Autodesk Inventor part; units mm, degrees
ref_plane "YZ Plane" through (0, 0, 0) normal (1, 0, 0) x (0, 1, 0)
ref_plane "XZ Plane" through (0, 0, 0) normal (0, 1, 0) x (-1, 0, 0)
ref_plane "XY Plane" through (0, 0, 0) normal (0, 0, 1) x (1, 0, 0)
sketch "Sketch1" plane through (0, 0, 0) normal (1, 0, 0) x (0, 1, 0)
  line L0 (64.7557, 308.0174) -> (-36.8443, 308.0174)
  line L1 (-36.8443, 308.0174) -> (-36.8443, -314.2826)
  line L2 (-36.8443, -314.2826) -> (64.7557, -314.2826)
  line L3 (64.7557, -314.2826) -> (64.7557, 308.0174)
  dimension "d2" = 622.3
  dimension "d3" = 101.6
extrude "Board" add sketch "Sketch1" along normal blind 19.05
sketch "Sketch8" plane through (19.05, 0, 0) normal (1, 0, 0) x (0, 0, -1)
  line L0 (-308.0174, 55.2307) -> (314.2826, 55.2307)
  line L1 (314.2826, 55.2307) -> (314.2826, 45.7057)
  line L2 (314.2826, 45.7057) -> (-308.0174, 45.7057)
  line L3 (-308.0174, 45.7057) -> (-308.0174, 55.2307)
  line L4 (-308.0174, 64.7557) -> (-308.0174, -36.8443)
  line L5 (314.2826, -36.8443) -> (314.2826, 64.7557)
  line L6 (314.2826, 64.7557) -> (-308.0174, 64.7557)
  point P0 (0, 0)
  dimension "d22" = 9.525
  dimension "d23" = 9.525
extrude "Lenghtwise Dado for Base" cut sketch "Sketch8" against normal blind 9.525 contours L0 L1 L2 L3
sketch "Sketch 9" plane through (0, 64.7557, 308.0174) normal (0, 1, 0) x (1, 0, 0)
  line L0 (19.05, 168.275) -> (9.525, 168.275)
  line L1 (9.525, 168.275) -> (9.525, 622.3)
  line L2 (9.525, 622.3) -> (19.05, 622.3)
  line L3 (19.05, 622.3) -> (19.05, 168.275)
  line L4 (19.05, 622.3) -> (19.05, 0)
  line L5 (0, 622.3) -> (19.05, 622.3)
  point P0 (0, 308.0174)
  dimension "d26" = 454.025
  dimension "d27" = 9.525
extrude "Lengthwise stop dado for Sides" cut sketch "Sketch 9" against normal blind 9.525
sketch "Sketch12" plane through (19.05, 0, 0) normal (1, 0, 0) x (0, 0, -1)
  line L0 (-308.0174, 64.7557) -> (-308.0174, -36.8443)
  line L1 (314.2826, -36.8443) -> (314.2826, 45.7057)
  line L2 (-308.0174, 46.2852) -> (314.2826, 46.2852)
  line L3 (314.2826, 46.2852) -> (314.2826, 27.2352)
  line L4 (314.2826, 27.2352) -> (-308.0174, 27.2352)
  line L5 (-308.0174, 27.2352) -> (-308.0174, 46.2852)
  dimension "d39" = 19.05
extrude "Extrusion10" cut sketch "Sketch12" against normal blind 9.525
properties part number "Base Runner Side"
Model file for the job. Use its own axes, mm. A direction names the side the tool comes from. Coordinates: 2 decimals unless noted, no trailing zeros. Order: outer loops, then holes, each group sorted by start corner. A loop starts at its lowest first (then second) coordinate and runs counter-clockwise, first axis right, second up. Notation, with made-up numbers: (82, 53) -> (136, 53) arc R19 ccw to (136, 69) -> close; hole circle Ø5 at (-26, -17). An arc over 180 degrees is marked (long way). Answer as a JSON object with one key per item and string values. Group by question number.
1) Flat gauge pins, fed straight in: pin 1 (7.5 mm diameter, centred on x = 12.5, z = 82.5, fed in from +Y); pin 2 (3 mm diameter, centred on x = 15, z = -151.5, fed in from +Y); pin 3 (5 mm diameter, centred on x = 13.5, y = 62, fed in from -Z). Where does each tip first touch, or does it go through?
2) Cut at A-A, the plane x = 14. Write the cut outline in (y, z), then the cut area to 3 significant figures.
3) Cut at C-C, the plane y = 32.5. Write the cut outline in (x, z) (3 decimals), then the cut area to 3 significant figures.
4) Pull direction Y, two halves, no side cores. Call faces 4 (the face through (19.05, 60, 225)), 5 (the face through (14, 55.231, 225)), 6 (the face through (9, -36.844, 1)): +Y half, -Y half, draft (parallel to the pull), parting line (faces both ways), or undercut.
5) Cut at B-B, the plane z = 146. Write the cut outline in (x, y) (3 decimals).
6) Drill centre lines: L1, parallel to X at y = 28, z = -200 (3 decimals); L2, parallel to Y at x = 12.5, z = -67. Where is each one in solid material? Low to high.
7) Which spindle directions (+Z, -Z, +X, -X, +Y, -Y) get a long thin tool onto all of the face, cutting with end or side? Do faces 1 (the face through (14, 27.235, -7)), 2 (the face through (14, 60, 139.742)), 3 (the face through (7, 64.756, 62)). Say none if no direction does.
Check values:
{
 "1": {"pin 1": "stops at y = 64.76", "pin 2": "stops at y = 27.24", "pin 3": "stops at z = 139.74"},
 "2": {"outline": "(-36.84, -314.28) -> (27.24, -314.28) -> (27.24, 308.02) -> (-36.84, 308.02) -> close; (55.23, 139.74) -> (64.76, 139.74) -> (64.76, 308.02) -> (55.23, 308.02) -> close", "area": "41,500 mm²"},
 "3": {"outline": "(0, -314.283) -> (9.525, -314.283) -> (9.525, 308.017) -> (0, 308.017) -> close", "area": "5,930 mm²"},
 "4": {"face 4": "draft", "face 5": "undercut", "face 6": "-Y half"},
 "5": {"outline": "(0, -36.844) -> (19.05, -36.844) -> (19.05, 27.235) -> (9.525, 27.235) -> (9.525, 55.231) -> (19.05, 55.231) -> (19.05, 64.756) -> (0, 64.756) -> close"},
 "6": {"L1": "x = 0 to 9.525", "L2": "y = -36.84 to 27.24"},
 "7": {"face 1": "+Z, -Z, +X", "face 2": "-Z, +X, +Y", "face 3": "+Z, -Z, +X, -X, +Y"}
}
